Check sheet for the modelled part. Datum: model origin and axes. Units: mm. A direction names the side the tool comes from. Give positions to 0.01 mm unless a question says otherwise; leave off trailing zeros. Order: outer loops, then holes, each group sorted by start corner. A loop starts at its lowest first (then second) coordinate and runs counter-clockwise, first axis right, second up.
from build123d import *

# Parameters (mm, degrees)
AUFSATZ_LINEAR_AUSTRAGEN1_DEPTH = 55.4
AUFSATZ_LINEAR_AUSTRAGEN2_DEPTH = 2.6
SCHNITT_LINEAR_AUSTRAGEN1_DEPTH = 7.5
SKIZZE4_R                       = 2.2
SCHNITT_LINEAR_AUSTRAGEN2_DEPTH = 10


with BuildPart() as part:
    # Skizze1 → Aufsatz-Linear austragen1 (new body)
    with BuildSketch(Plane(origin=(0, 0, 0), x_dir=(1, 0, 0), z_dir=(0, 1, 0))):
        with BuildLine():
            Line((137.5, 238.156986041), (145, 251.147367097))
            ThreePointArc((145, 251.147367097), (251.147367097, 145), (290, 0))
            Line((290, 0), (275, 0))
            ThreePointArc((275, 0), (238.156986041, 137.5), (137.5, 238.156986041))
        make_face()
    extrude(amount=AUFSATZ_LINEAR_AUSTRAGEN1_DEPTH)

    # Skizze2 → Aufsatz-Linear austragen2 (add)
    with BuildSketch(Plane(origin=(0, 55.4, 0), x_dir=(1, 0, 0), z_dir=(0, 1, 0))):
        with BuildLine():
            Line((140.5, 243.353138463), (142, 245.951214675))
            ThreePointArc((142, 245.951214675), (245.951214675, 142), (284, 0))
            Line((284, 0), (281, 0))
            ThreePointArc((281, 0), (243.353138463, 140.5), (140.5, 243.353138463))
        make_face()
    extrude(amount=AUFSATZ_LINEAR_AUSTRAGEN2_DEPTH)

    # Skizze3 → Schnitt-Linear austragen1 (cut)
    with BuildSketch(Plane(origin=(0, 58, 0), x_dir=(1, 0, 0), z_dir=(0, 1, 0))):
        Polygon((269.165136135, 77.29896176), (273.994765267, 78.593056986), (276.582955718, 68.933798723), (271.753326586, 67.639703497), align=None)
        Polygon((194.454364826, 201.525432638), (197.989898732, 205.060966544), (205.060966544, 197.989898732), (201.525432638, 194.454364826), align=None)
    extrude(amount=-SCHNITT_LINEAR_AUSTRAGEN1_DEPTH, mode=Mode.SUBTRACT)

    # Skizze4 → Schnitt-Linear austragen2 (cut)
    with BuildSketch(Plane.XZ):
        with Locations(Location((199.757665685, -199.757665685, 0), (0, 0, 270))):
            Circle(SKIZZE4_R)
        with Locations(Location((272.874045927, -73.116380241, 0), (0, 0, 270))):
            Circle(SKIZZE4_R)
    extrude(amount=-SCHNITT_LINEAR_AUSTRAGEN2_DEPTH, mode=Mode.SUBTRACT)


solid = part.part
1) Section check B-B, the plane z = -102. Record the cut outline in (x, y), then the cut area to 3 significant figures.
Recorded:
outline: (255.38, 0) - (271.47, 0) - (271.47, 55.4) - (265.05, 55.4) - (265.05, 58) - (261.83, 58) - (261.83, 55.4) - (255.38, 55.4) - close
area: 900 mm2
2) Section check D-D, the plane y = 37.5. Record the cut outline in (x, z), then the cut area to 3 significant figures.
Recorded:
outline: (137.5, -238.16) - (145, -251.15) arc R290 ccw to (290, 0) - (275, 0) arc R275 cw to start
area: 4,440 mm2
3) Material ranges on L1, parallel to Y at x = 274.5, z = -25; L2, parallel to X at y = 40, z = -200; L3, parallel to Z at x = 184, y = 54.5, recorded low to high.
Recorded:
L1: y = 0 to 55.4
L2: x = 188.75 to 210
L3: z = -224.15 to -204.37
4) Section check C-C, the plane y = 7. Record the cut outline in (x, z).
Recorded:
outline: (137.5, -238.16) - (145, -251.15) arc R290 ccw to (290, 0) - (275, 0) arc R275 cw to start; hole circle Ø4.4 at (199.76, -199.76); hole circle Ø4.4 at (272.87, -73.12)
5) Draft check along Z on faces 1 (the face through (271.55, 53.47, -77.94)), 2 (the face through (170.51, 56.682, -227.117)), 3 (the face through (201.48, 52.98, -201.57)), 4 (the face through (283, 29, 0)). Enter one of: +Z half, -Z half, draft (parallel to the pull), parting line (faces both ways), or undercut.
Recorded:
face 1: undercut
face 2: -Z half
face 3: undercut
face 4: +Z half
6) Set-up check for faces 5 (the face through (169.45, 56.68, -224.16)), 6 (the face through (250.1, 27.3, -146.8)), 7 (the face through (281.826, 56.682, -35.071)), 8 (the face through (239.16, 27.31, -135.75)), 9 (the face through (274.202, 53.469, -68.296)): record each of +Z, -Z, +X, -X, +Y, -Y from which the full face is reachable in a straight line by a thin tool's end or side.
Recorded:
face 5: +Z, -X, +Y
face 6: -Z, +X, +Y, -Y
face 7: -Z, +X, +Y
face 8: +Z, -X, +Y, -Y
face 9: +Y
7) Depth check by flat-ended pin: pin 1 Ø2 at (x, z) = (272.5, -75) entering from +Y; pin 2 Ø10 at (y, z) = (23, -72) entering from +X; pin 3 Ø1 at (x, y) = (164, 29.5) entering from -Z. Enter the tip coordinate at first touch or a pass-through.
Recorded:
pin 1: stops at y = 50.5
pin 2: stops at x = 282.15
pin 3: stops at z = -239.52
8) Section check A-A, the plane x = 264.5. Record the cut outline in (y, z), then the cut area to 3 significant figures.
Recorded:
outline: (0, -118.91) - (55.4, -118.91) - (55.4, -103.42) - (58, -103.42) - (58, -94.87) - (55.4, -94.87) - (55.4, -75.26) - (0, -75.26) - close
area: 2,440 mm2
